from build123d import *

# Parameters (mm, degrees)
PAD_DEPTH    = 3.5
CHAMFER_SIZE = 0.275


with BuildPart() as part:
    # Sketch → Revolution (revolve)
    with BuildSketch(Plane(origin=(0, 0, 0), x_dir=(-1, 0, 0), z_dir=(0, 1, 0))):
        with BuildLine():
            Line((0, 0), (0.933333, 0))
            ThreePointArc((0.933333, 0), (0.980474, 0.019526), (1, 0.066667))
            Line((1, 0.066667), (1, 0.433333))
            ThreePointArc((1, 0.433333), (0.980474, 0.480474), (0.933333, 0.5))
            Line((0.933333, 0.5), (0.5, 0.5))
            Line((0.5, 0.5), (0.5, 6.375))
            ThreePointArc((0.5, 6.375), (0.463388, 6.463388), (0.375, 6.5))
            Line((0.375, 6.5), (0, 6.5))
            Line((0, 6.5), (0, 0))
        make_face()
    revolve(axis=Axis((0, 0, 0), (0, 0, 1)))

    # Sketch001 → Pad (new body)
    with BuildSketch(Plane.XY):
        Polygon((-0.55, 0), (0, 0.55), (0.55, 0), (0, -0.55), align=None)
    extrude(amount=-PAD_DEPTH)

    # Chamfer
    chamfer_edges = [part.edges().sort_by_distance(p)[0] for p in [
        (0.275, -0.275, -3.5),
        (-0.275, -0.275, -3.5),
        (-0.275, 0.275, -3.5),
        (0.275, 0.275, -3.5),
    ]]
    chamfer(chamfer_edges, length=CHAMFER_SIZE)


solid = part.part
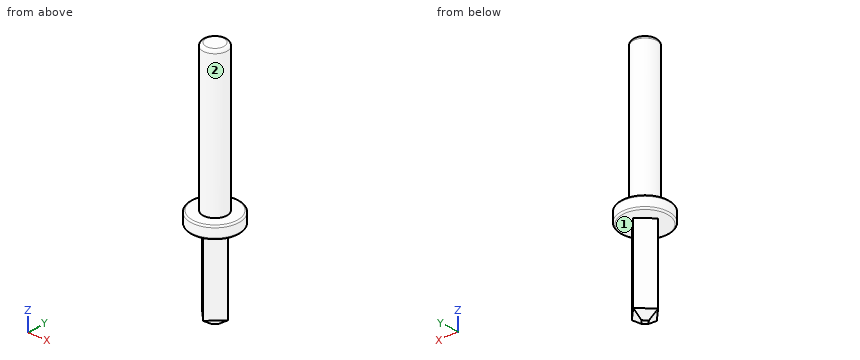
Build history of the part. All positions in model axes, mm. Face numbers are marked on the shaded views. A direction names the side the tool comes from. Round coordinates to 2 decimals unless told otherwise and drop trailing zeros. Loops run counter-clockwise (first coordinate to the right, second up) from the corner with the lowest first, then second, coordinate; pieces in that order, holes last. Notation, with made-up numbers: (21, -24) -> (31, -24) arc R20 ccw to (31, -20) -> close; hole circle Ø2 at (-2, -21). An arc over 180 degrees is marked (long way). One line per item, written item: value. Start each with the question number.
Q1. Cut at B-B on z = 2.75. List the corners of the cut face in (x, y), plus the area to 3 significant figures.
Q2. 3-axis set-ups, long thin cutter, end or side, ignore diameter. For the marked faces 1 and 2: which of +Z, -Z, +X, -X, +Y, -Y reach the whole face in a straight line?
Q3. Drop flat-ended pins along their axis: pin 1 Ø0.9 at (x, y) = (-0.5, 0.5) entering from -Z; pin 2 Ø1 at (x, z) = (0, -1.5) entering from +Y. Give the stop position or say it passes through.
Q4. Probe line 1 along Z through (x, y) = (-0.7, -0.45); line 2 along X through (y, z) = (-0.05, 3.5); line 3 along X through (y, z) = (0.15, -1.75). List the from-to ranges inside material, lowest first.
Q5. Cut at A-A on z = -3. List the corners of the cut face in (x, y).
Computed:
1. outline: circle Ø1 at (0, 0)
1. area: 0.785 mm²
2. face 1: -Z
2. face 2: +Z
3. pin 1: z = -3.36
3. pin 2: y = 0.55
4. line 1: 0 to 0.5
4. line 2: -0.5 to 0.5
4. line 3: -0.4 to 0.4
5. outline: (-0.55, 0) -> (0, -0.55) -> (0.55, 0) -> (0, 0.55) -> close
